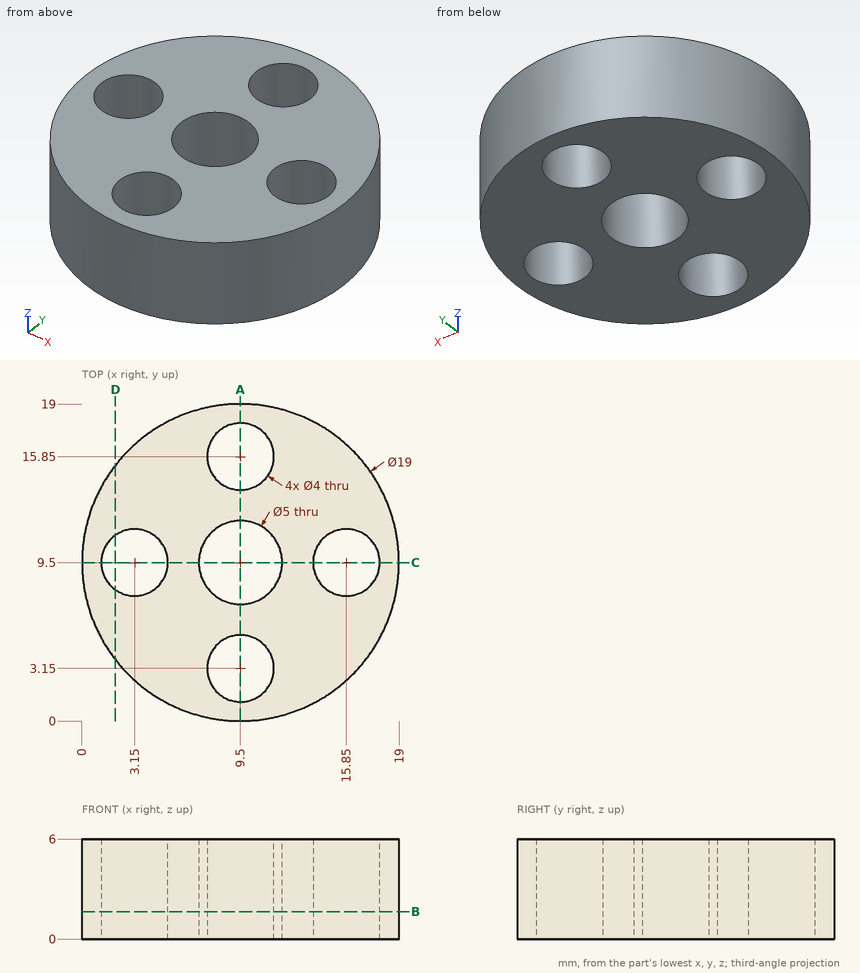
Geometry check sheet. Reference: drawing and pictorial views, mm from the part's lowest x, y, z. Coordinates: 2 decimals unless noted, no trailing zeros. Order: outer loops, then holes, each group sorted by start corner. A loop starts at its lowest first (then second) coordinate and runs counter-clockwise, first axis right, second up. Notation, with made-up numbers: (69, 9) -> (122, 9) arc R34 ccw to (122, 47) -> close; hole circle Ø11 at (84.25, -26.5). An arc over 180 degrees is marked (long way). Use CSV: the item, a comma, the result in double quotes. Start each with the question number.
Q1. Section check A-A, the plane x = 9.5. Record the cut outline in (y, z), and give its area (3 significant figures).
Q2. Thickness scan on line 1 along Y through (x, z) = (9.5, 3.45); line 2 along Y through (x, z) = (10, 5.25). Record the ranges inside material, lowest first.
Q3. Depth check by flat-ended pin: P1, Ø4, axis at x = 11, y = 16, coming from the -Z side; P2, Ø3.5, axis at x = 9.5, y = 3.15, coming from the -Z side; P3, Ø2, axis at x = 4.5, z = 3, coming from the -Y side; P4, Ø1, axis at y = 12, z = 2.5, coming from the -X side. Enter the tip coordinate at first touch or a pass-through.
Q4. Section check B-B, the plane z = 1.65. Record the cut outline in (x, y), and give its area (3 significant figures).
Q5. Section check D-D, the plane x = 2. Record the cut outline in (y, z), and give its area (3 significant figures).
Returned:
1,outline,"(0, 0) -> (1.15, 0) -> (1.15, 6) -> (0, 6) -> close; (5.15, 0) -> (7, 0) -> (7, 6) -> (5.15, 6) -> close; (12, 0) -> (13.85, 0) -> (13.85, 6) -> (12, 6) -> close; (17.85, 0) -> (19, 0) -> (19, 6) -> (17.85, 6) -> close"
1,area,"36.0 mm^2"
2,line 1,"y = 0 to 1.15, 5.15 to 7, 12 to 13.85, 17.85 to 19"
2,line 2,"y = 0.01 to 1.21, 5.09 to 7.05, 11.95 to 13.91, 17.79 to 18.99"
3,P1,"stops at z = 0"
3,P2,"passes through"
3,P3,"stops at y = 0.88"
3,P4,"stops at x = 0.21"
4,outline,"circle Ø19 at (9.5, 9.5); hole circle Ø4 at (3.15, 9.5); hole circle Ø5 at (9.5, 9.5); hole circle Ø4 at (9.5, 3.15); hole circle Ø4 at (9.5, 15.85); hole circle Ø4 at (15.85, 9.5)"
4,area,"214 mm^2"
5,outline,"(3.67, 0) -> (7.86, 0) -> (7.86, 6) -> (3.67, 6) -> close; (11.14, 0) -> (15.33, 0) -> (15.33, 6) -> (11.14, 6) -> close"
5,area,"50.3 mm^2"
